Geometry: final body of the model. Coordinates: model frame, mm. Give positions to 0.01 mm unless a question says otherwise; leave off trailing zeros. Write each loop counter-clockwise with the first axis right and the second up, starting at its lowest first coordinate (ties: lowest second). Pieces come first, ordered by that corner, then holes. Notation, with made-up numbers: M 59,-15 L 65,-15 A17 cw 65,-1 Z; hole C 66,10.25 d6. An arc over 180 degrees is marked long. Answer as a JSON object with one key per item and string values.
from build123d import *

# Parameters (mm, degrees)
F0_W     = 50.8
F0_H     = 76.2
F1_DEPTH = 25.4
F3_D     = 6.35
F4_R     = 5.08


with BuildPart() as f1:
    # F0 (on Front) → F1 (new body)
    with BuildSketch(Plane.XZ):
        with Locations((25.4, 38.1)):
            Rectangle(F0_W, F0_H)
    extrude(amount=F1_DEPTH)

    # F3 (through all)
    with Locations(Plane.XZ.offset(25.4)):
        with Locations((16.642079, 18.818352)):
            Hole(F3_D / 2)

    # F4
    f4_edges = [f1.edges().sort_by_distance(p)[0] for p in [
        (0, -25.4, 38.1),
        (25.4, -25.4, 76.2),
        (25.4, -25.4, 0),
        (50.8, -25.4, 38.1),
        (13.467079, -25.4, 18.818352),
    ]]
    fillet(f4_edges, radius=F4_R)


solid = f1.part
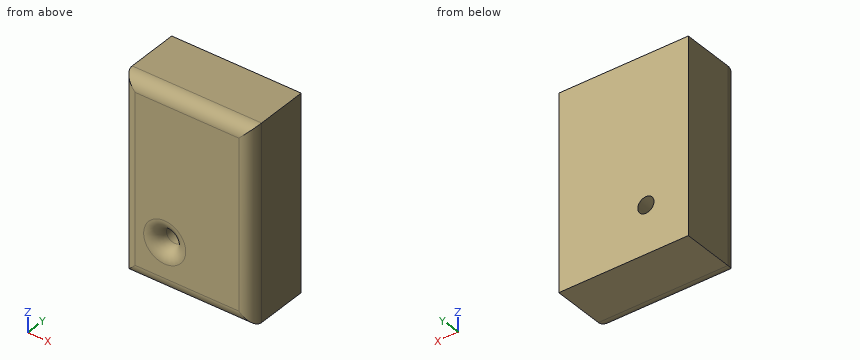
1) Cut plane A-A on y = -23. Return loops of the section in (x, z), and give its area (3 significant figures).
Geometry check:
{"outline": "M 0.76,0.76 L 50.04,0.76 L 50.04,75.44 L 0.76,75.44 Z; hole C 16.64,18.82 d7.88", "area": "3,630 mm2"}
2) Contact query for flat-ended pins moving along their axis: P1, Ø1.5, axis at y = -22, z = 46, coming from the +X side; P2, Ø5, axis at x = 16.64, z = 18.82, coming from the +Y side. Output: stop coordinate, or through.
Geometry check:
{"P1": "stops at x = 50.71", "P2": "passes through"}
3) Line query: line 1 (Z direction, x = 14, y = -18.5); line 2 (X direction, y = -22.75, z = 71.5); line 3 (Z direction, x = 27, y = -21.25). Output: solid intervals per line, ascending. Write a range as from..to.
Geometry check:
{"line 1": "z = 0..17.06, 20.58..76.2", "line 2": "x = 0.62..50.18", "line 3": "z = 0.09..76.11"}
